from build123d import *

# Parameters (mm, degrees)
SKETCH1_W           = 170
SKETCH1_H           = 100
BOSS_EXTRUDE1_DEPTH = 45
SKETCH3_W           = 30
SKETCH3_H           = 98
CUT_EXTRUDE2_DEPTH  = 18
SKETCH4_W           = 30
SKETCH4_H           = 10
SKETCH4_H_2         = 15
CUT_EXTRUDE3_DEPTH  = 15
SKETCH5_R           = 1.5
CUT_EXTRUDE4_DEPTH  = 3


with BuildPart() as part:
    # Sketch1 → Boss-Extrude1 (new body)
    with BuildSketch(Plane.XY):
        with Locations((76.199255121, -45.298882682)):
            Rectangle(SKETCH1_W, SKETCH1_H)
    extrude(amount=BOSS_EXTRUDE1_DEPTH)

    # Sketch3 → Cut-Extrude2 (cut)
    with BuildSketch(Plane.XY.offset(45)):
        with Locations((146.199255121, -46.298882682)):
            Rectangle(SKETCH3_W, SKETCH3_H)
    extrude(amount=-CUT_EXTRUDE2_DEPTH, mode=Mode.SUBTRACT)

    # Sketch4 → Cut-Extrude3 (cut)
    with BuildSketch(Plane.XY.offset(27)):
        with Locations((146.199255121, -90.298882682)):
            Rectangle(SKETCH4_W, SKETCH4_H)
        with Locations((146.199255121, -4.798882682)):
            Rectangle(SKETCH4_W, SKETCH4_H_2)
    extrude(amount=-CUT_EXTRUDE3_DEPTH, mode=Mode.SUBTRACT)

    # Sketch5 → Cut-Extrude4 (cut)
    with BuildSketch(Plane(origin=(0, 4.701117318, 0), x_dir=(1, 0, 0), z_dir=(0, 1, 0))):
        with Locations(Location((-5.800744879, -32, 0), (0, 0, 270))):
            Circle(SKETCH5_R)
        with Locations(Location((144.199255121, -32, 0), (0, 0, 270))):
            Circle(SKETCH5_R)
    extrude(amount=-CUT_EXTRUDE4_DEPTH, mode=Mode.SUBTRACT)


solid = part.part
The listing builds one solid part. Answer for the finished solid, in the listing's coordinates (mm). A direction names the side the tool comes from. Coordinates: 2 decimals unless noted, no trailing zeros. Loops run counter-clockwise (first coordinate to the right, second up) from the corner with the lowest first, then second, coordinate; pieces in that order, holes last. Notation, with made-up numbers: M 53.5,-13.5 L 72.5,-13.5 A35 ccw 72.5,23.5 Z; hole C 67,32.25 d8. An arc over 180 degrees is marked long. Answer in a Markdown table with one row per item.
1) Which of the six approach directions +Z, -Z, +X, -X, +Y, -Y give full straight-line access (tool end or side, diameter ignored) to faces 4 (the flat face through (146, -90, 12)), 5 (the flat face through (146, -12.299, 20)), 6 (the flat face through (-8.801, -46, 22))?
Answers below:
| item | result |
|---|---|
| face 4 | +Z, +X, -Y |
| face 5 | +Z, +X |
| face 6 | +Z, -Z, -X, +Y, -Y |
2) Find section B-B (z = 17.5). Determine the outline of the cut face in (x, y), then the cut area to 4 significant figures.
Answers below:
| item | result |
|---|---|
| outline | M -8.8,-95.3 L 131.2,-95.3 L 131.2,-85.3 L 161.2,-85.3 L 161.2,-12.3 L 131.2,-12.3 L 131.2,2.7 L 161.2,2.7 L 161.2,4.7 L -8.8,4.7 Z |
| area | 16,250 mm^2 |
3) Find section A-A (y = -78). Determine the outline of the cut face in (x, z), then the cut area to 3 significant figures.
Answers below:
| item | result |
|---|---|
| outline | M -8.8,0 L 161.2,0 L 161.2,27 L 131.2,27 L 131.2,45 L -8.8,45 Z |
| area | 7,110 mm^2 |
4) Find the intervals of material crossed by probe 1 along X at (y, z) = (3.85, 32); probe 2 along X at (y, z) = (-15.5, 42); probe 3 along X at (y, z) = (2.65, 32), in increasing order.
Answers below:
| item | result |
|---|---|
| probe 1 | -8.8 to -7.3, -4.3 to 142.7, 145.7 to 161.2 |
| probe 2 | -8.8 to 131.2 |
| probe 3 | -8.8 to -7.3, -4.3 to 131.2 |
5) Given pin 1 (5 mm diameter, centred on x = 143.5, y = -88, fed in from +Z); pin 2 (3.5 mm diameter, centred on x = -5.5, z = 32, fed in from +Y); pin 3 (3.5 mm diameter, centred on x = 144.2, z = 32, fed in from -Y); pin 4 (9 mm diameter, centred on x = 149.5, y = -46.5, fed in from +Z), each flat-ended and moving along its own axis, determine where each tip first touches the part or whether it passes through.
Answers below:
| item | result |
|---|---|
| pin 1 | z = 12 |
| pin 2 | y = 4.7 |
| pin 3 | y = 2.7 |
| pin 4 | z = 27 |
6) Find section C-C (z = 40). Determine the outline of the cut face in (x, y).
Answers below:
| item | result |
|---|---|
| outline | M -8.8,-95.3 L 131.2,-95.3 L 131.2,2.7 L 161.2,2.7 L 161.2,4.7 L -8.8,4.7 Z |
7) Determine the mould class of faces 1 (the flat face through (75, -45, 0)), 2 (the flat face through (75, 4.701, 22)), 3 (the flat face through (146, -5, 12)) for opening direction Y: released by +Y, released by -Y, zero draft, split by the parting line, or undercut.
Answers below:
| item | result |
|---|---|
| face 1 | zero draft |
| face 2 | released by +Y |
| face 3 | undercut |
